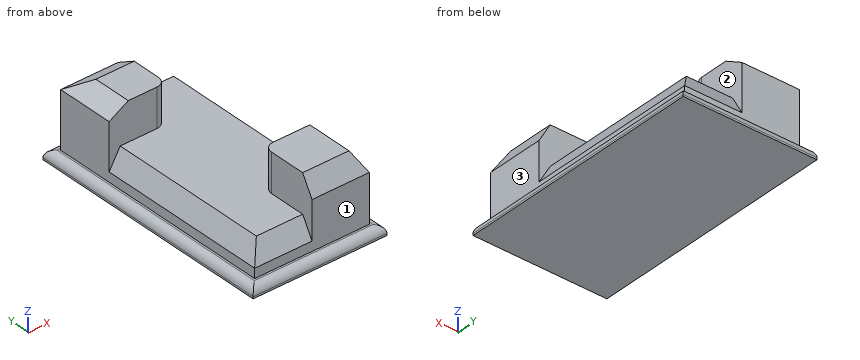
```python
from build123d import *

# Parameters (mm, degrees)
F1_DEPTH    = 25.4
F2_DEPTH    = 50.8
F0_W        = 88.9
F0_H        = 165.1
F3_DEPTH    = 6.35
F4_R        = 5.08
F5_SIZE2    = 7.3323484187
F5_SIZE     = 12.7
F6_C1_SIZE2 = 12.7
F6_C1_SIZE  = 7.3323484187
F6_C2_SIZE2 = 7.3323484187
F6_C2_SIZE  = 12.7
F6_C3_SIZE2 = 12.7
F6_C3_SIZE  = 7.3323484187
F6_C4_SIZE2 = 7.3323484187
F6_C4_SIZE  = 12.7


with BuildPart() as f1:
    # F0 (on Top) → F1 (new body)
    with BuildSketch(Plane.XY):
        with BuildLine():
            Line((-19.5483354544, 60.1456080113), (-51.2983354544, 60.1456080113))
            Line((-51.2983354544, 60.1456080113), (-51.2983354544, -54.1543919887))
            Line((-51.2983354544, -54.1543919887), (-13.1983354544, -54.1543919887))
            Line((-13.1983354544, -54.1543919887), (-13.1983354544, -22.4043919887))
            ThreePointArc((-13.1983354544, -22.4043919887), (-11.3384635149, -17.9142639282), (-6.8483354544, -16.0543919887))
            Line((-6.8483354544, -16.0543919887), (24.9016645456, -16.0543919887))
            Line((24.9016645456, -16.0543919887), (24.9016645456, 98.2456080113))
            Line((24.9016645456, 98.2456080113), (-13.1983354544, 98.2456080113))
            Line((-13.1983354544, 98.2456080113), (-13.1983354544, 66.4956080113))
            ThreePointArc((-13.1983354544, 66.4956080113), (-15.0582073938, 62.0054799508), (-19.5483354544, 60.1456080113))
        make_face()
    extrude(amount=F1_DEPTH)

    # F0 (on Top) → F2 (join)
    with BuildSketch(Plane.XY):
        with BuildLine():
            Line((-13.1983354544, 98.2456080113), (-51.2983354544, 98.2456080113))
            Line((-51.2983354544, 98.2456080113), (-51.2983354544, 60.1456080113))
            Line((-51.2983354544, 60.1456080113), (-19.5483354544, 60.1456080113))
            ThreePointArc((-19.5483354544, 60.1456080113), (-15.0582073938, 62.0054799508), (-13.1983354544, 66.4956080113))
            Line((-13.1983354544, 66.4956080113), (-13.1983354544, 98.2456080113))
        make_face()
        with BuildLine():
            Line((-13.1983354544, -22.4043919887), (-13.1983354544, -54.1543919887))
            Line((-13.1983354544, -54.1543919887), (24.9016645456, -54.1543919887))
            Line((24.9016645456, -54.1543919887), (24.9016645456, -16.0543919887))
            Line((24.9016645456, -16.0543919887), (-6.8483354544, -16.0543919887))
            ThreePointArc((-6.8483354544, -16.0543919887), (-11.3384635149, -17.9142639282), (-13.1983354544, -22.4043919887))
        make_face()
    extrude(amount=F2_DEPTH)

    # F0 (on Top) → F3 (join)
    with BuildSketch(Plane.XY):
        with Locations((-13.1983354544, 22.0456080113)):
            Rectangle(F0_W, F0_H)
        Polygon((-51.2983354544, 60.1456080113), (-51.2983354544, 98.2456080113), (-13.1983354544, 98.2456080113), (24.9016645456, 98.2456080113), (24.9016645456, -16.0543919887), (24.9016645456, -54.1543919887), (-13.1983354544, -54.1543919887), (-51.2983354544, -54.1543919887), align=None, mode=Mode.SUBTRACT)
    extrude(amount=F3_DEPTH)

    # F4
    f4_edges = [f1.edges().sort_by_distance(p)[0] for p in [
        (31.251665, 22.045608, 6.35),
        (-13.198335, -60.504392, 6.35),
        (-57.648335, 22.045608, 6.35),
        (-13.198335, 104.595608, 6.35),
    ]]
    fillet(f4_edges, radius=F4_R)

    # F5
    f5_edges = [f1.edges().sort_by_distance(p)[0] for p in [
        (24.901665, 41.095608, 25.4),
        (5.851665, 98.245608, 25.4),
        (-51.298335, 2.995608, 25.4),
        (-32.248335, -54.154392, 25.4),
    ]]
    chamfer(f5_edges, length=F5_SIZE, length2=F5_SIZE2)

    # F6: chamfer of 12.7 x 7.3323484187 on 4 edges, made by hand

    # F6_c1
    f6_c1_edges = [f1.edges().sort_by_distance(p)[0] for p in [
        (-51.2983354544, 79.1956080113, 50.8),
    ]]
    f6_c1_side = f1.faces().sort_by_distance((-51.2983354544, 79.1956080113, 50.6533530316))[0]
    chamfer(f6_c1_edges, length=F6_C1_SIZE, length2=F6_C1_SIZE2, reference=f6_c1_side)

    # F6_c2
    f6_c2_edges = [f1.edges().sort_by_distance(p)[0] for p in [
        (5.8516645456, -54.1543919887, 50.8),
    ]]
    f6_c2_side = f1.faces().sort_by_distance((5.8516645456, -54.1543919887, 50.6533530316))[0]
    chamfer(f6_c2_edges, length=F6_C2_SIZE, length2=F6_C2_SIZE2, reference=f6_c2_side)

    # F6_c3
    f6_c3_edges = [f1.edges().sort_by_distance(p)[0] for p in [
        (-25.8983354544, 98.2456080113, 50.8),
    ]]
    f6_c3_side = f1.faces().sort_by_distance((-25.8983354544, 98.2456080113, 50.6533530316))[0]
    chamfer(f6_c3_edges, length=F6_C3_SIZE, length2=F6_C3_SIZE2, reference=f6_c3_side)

    # F6_c4
    f6_c4_edges = [f1.edges().sort_by_distance(p)[0] for p in [
        (24.9016645456, -31.4382177794, 50.8),
    ]]
    f6_c4_side = f1.faces().sort_by_distance((24.9016645456, -31.4382177794, 50.6533530316))[0]
    chamfer(f6_c4_edges, length=F6_C4_SIZE, length2=F6_C4_SIZE2, reference=f6_c4_side)


solid = f1.part
```
Build history of the part. All positions in model axes, mm. Face numbers are marked on the shaded views. A direction names the side the tool comes from. Give positions to 0.01 mm unless a question says otherwise; leave off trailing zeros. Loops run counter-clockwise (first coordinate to the right, second up) from the corner with the lowest first, then second, coordinate; pieces in that order, holes last. Notation, with made-up numbers: (-7.5, -21) -> (2.5, -21) arc R21 ccw to (2.5, -11) -> close; hole circle Ø10 at (26.25, 65.25). An arc over 180 degrees is marked (long way). One line per question, with ' | ' between items.
Q1. Drill centre lines: line 1 along Z through (x, y) = (-40.5, 57.5); line 2 along Y through (x, z) = (-41.5, 7); line 3 along X through (y, z) = (42, 8). Where is each one in solid material? Low to high. Write a range as [from, to].
Filled sheet:
line 1: z = [0, 25.4] | line 2: y = [-54.15, 98.25] | line 3: x = [-51.3, 24.9]
Q2. Cut at A-A, the plane z = 45.5. Write the cut outline in (x, y), plus the area to 3 significant figures.
Filled sheet:
outline: (-47.78, 60.15) -> (-19.55, 60.15) arc R6.35 ccw to (-13.2, 66.5) -> (-13.2, 94.73) -> (-47.78, 94.73) -> close; (-13.2, -49.88) -> (20.63, -49.88) -> (20.63, -16.05) -> (-6.85, -16.05) arc R6.35 ccw to (-13.2, -22.4) -> close | area: 2,320 mm²
Q3. Drop flat-ended pins along their axis: pin 1 (2 mm diameter, centred on y = 12.5, z = 21.5, fed in from -X) (3 decimals); pin 2 (12 mm diameter, centred on x = -41, z = 39, fed in from +Y); pin 3 (5 mm diameter, centred on x = -47.5, z = 25, fed in from -Y). Give the stop position or say it passes through.
Filled sheet:
pin 1: stops at x = -46.795 | pin 2: stops at y = 98.25 | pin 3: stops at y = 60.15
Q4. Cut at D-D, the plane z = 21. Write the cut outline in (x, y), plus the area to 3 significant figures.
Filled sheet:
outline: (-51.3, 60.15) -> (-46.51, 60.15) -> (-46.51, -49.36) -> (-13.2, -49.36) -> (-13.2, -54.15) -> (24.9, -54.15) -> (24.9, -16.05) -> (20.11, -16.05) -> (20.11, 93.45) -> (-13.2, 93.45) -> (-13.2, 98.25) -> (-51.3, 98.25) -> close | area: 10,200 mm²
Q5. Tool access for the marked faces 1, 2 and 3: list every direction of +Z, -Z, +X, -X, +Y, -Y with a clear straight run to the whole face (end or side of a thin tool).
Filled sheet:
face 1: +Z, +X, -X, -Y | face 2: +Z, +X, +Y | face 3: +Z, +X, +Y, -Y
Q6. Cut at B-B, the plane y = 26. Write the cut outline in (x, z).
Filled sheet:
outline: (-57.65, 0) -> (31.25, 0) -> (31.25, 1.27) arc R5.08 ccw to (26.17, 6.35) -> (24.9, 6.35) -> (24.9, 12.7) -> (17.57, 25.4) -> (-43.97, 25.4) -> (-51.3, 12.7) -> (-51.3, 6.35) -> (-52.57, 6.35) arc R5.08 ccw to (-57.65, 1.27) -> close
Q7. Cut at C-C, the plane x = 23. Write the cut outline in (y, z), plus the area to 3 significant figures.
Filled sheet:
outline: (-60.5, 0) -> (104.6, 0) -> (104.6, 1.27) arc R5.08 ccw to (99.52, 6.35) -> (98.25, 6.35) -> (98.25, 12.7) -> (96.34, 15.99) -> (-16.05, 15.99) -> (-16.05, 41.39) -> (-52.25, 41.39) -> (-54.15, 38.1) -> (-54.15, 6.35) -> (-55.42, 6.35) arc R5.08 ccw to (-60.5, 1.27) -> close | area: 3,470 mm²
